Autodesk Inventor part; units mm, degrees
ref_plane "YZ Plane" through (0, 0, 0) normal (1, 0, 0) x (0, 1, 0)
ref_plane "XZ Plane" through (0, 0, 0) normal (0, 1, 0) x (-1, 0, 0)
ref_plane "XY Plane" through (0, 0, 0) normal (0, 0, 1) x (1, 0, 0)
sketch "Sketch2" plane through (0, 0, 0) normal (1, 0, 0) x (0, 1, 0)
  line L0 (0, 0) -> (17, 0)
  line L1 (17, 0) -> (17, -15)
  line L2 (17, -15) -> (0, -15)
  line L3 (0, -15) -> (0, 0)
  dimension "d4" = 17
  dimension "d5" = 15
extrude "Extrusion2" add sketch "Sketch2" along normal blind 165
sketch "Sketch3" plane through (165, 0, 0) normal (1, 0, 0) x (0, 0, -1)
  line L0 (0, 17) -> (0, 0)
  line L1 (0, 0) -> (15, 0)
  line L2 (15, 0) -> (15, 17)
  line L3 (2, 2) -> (13, 2)
  line L4 (13, 2) -> (13, 15)
  line L5 (13, 15) -> (2, 15)
  line L6 (2, 15) -> (2, 2)
  line L7 (2, 2) -> (13, 15) construction
  line L8 (13, 2) -> (2, 15) construction
  point P0 (7.5, 8.5)
  dimension "d9" = 11
  dimension "d10" = 13
extrude "Extrusion3" cut sketch "Sketch3" against normal through all
sketch "Sketch5" plane through (0, 0, -15) normal (0, 0, -1) x (-1, 0, 0)
  line L0 (0, 0) -> (-165, 0)
  line L1 (-165, 0) -> (0, 17)
  line L2 (-165, 0) -> (-165, 17)
  line L3 (0, 0) -> (-165, 17)
  circle A0 centre (-82.5, 8.5) radius 4.5
  dimension "d13" = 9
extrude "Extrusion4" cut sketch "Sketch5" against normal through all contours A0 L1 L3 | L3 L1 A0 | A0 L3 L1 | L3 A0 L1
fillet "Fillet1" radius 1 4 edges at (82.5, 2, -13) (82.5, 2, -2) (82.5, 15, -2) (82.5, 15, -13)
properties part number "caja perfil"
Geometry: final body of the model. Coordinates: model frame, mm. A direction names the side the tool comes from. Give positions to 0.01 mm unless a question says otherwise; leave off trailing zeros. Write each loop counter-clockwise with the first axis right and the second up, starting at its lowest first coordinate (ties: lowest second). Pieces come first, ordered by that corner, then holes. Notation, with made-up numbers: (-20.75, 22.25) -> (-12.75, 22.25) arc R9 cw to (-12.75, 34.25) -> close; hole circle Ø3 at (79, 6.5). An arc over 180 degrees is marked (long way). Answer in a Markdown table with one row per item.
(1) Pin query (flat end, axial travel): pin 1 (8 mm diameter, centred on y = 14.5, z = -10.5, fed in from +X). Return the tip coordinate at first contact, or that it passes through.
Answers below:
| item | result |
|---|---|
| pin 1 | x = 165 |
(2) Draft query along Y for faces 1 (the flat face through (81, 17, -7)), 2 (the flat face through (81, 14, -15)), 3 (the flat face through (84, 4, -2)). Return one class per face: +Y half, -Y half, draft (parallel to the pull), parting line (faces both ways), or undercut.
Answers below:
| item | result |
|---|---|
| face 1 | +Y half |
| face 2 | draft |
| face 3 | undercut |
(3) Section query D-D on x = 28.5. Return loops of the section in (y, z).
Answers below:
| item | result |
|---|---|
| outline | (0, -15) -> (17, -15) -> (17, 0) -> (0, 0) -> close; hole (2, -12) arc R1 ccw to (3, -13) -> (14, -13) arc R1 ccw to (15, -12) -> (15, -3) arc R1 ccw to (14, -2) -> (3, -2) arc R1 ccw to (2, -3) -> close |
(4) Set-up query: faces 4 (the flat face through (0, 8, -1)), 5 (the flat face through (84, 15, -8)). Return all of +Z, -Z, +X, -X, +Y, -Y with unobstructed straight access to the full face (end or side cutting, diameter ignored); none if empty.
Answers below:
| item | result |
|---|---|
| face 4 | +Z, -Z, -X, +Y, -Y |
| face 5 | +X, -X |
(5) Section query B-B on z = -9.75. Return loops of the section in (x, y).
Answers below:
| item | result |
|---|---|
| outline | (0, 0) -> (165, 0) -> (165, 2) -> (0, 2) -> close; (0, 15) -> (165, 15) -> (165, 17) -> (0, 17) -> close |
(6) Ray query, line 1 along Z through (x, y) = (18.5, 4.25); line 2 along Y through (x, z) = (82.5, -0.7); line 3 along X through (y, z) = (8.5, -13.45). Return the intervals inside material, ascending. Write a range as [from, to].
Answers below:
| item | result |
|---|---|
| line 1 | [-15, -13], [-2, 0] |
| line 2 | [0, 4], [13, 17] |
| line 3 | [0, 78], [87, 165] |
(7) Section query A-A on y = 8.5. Return loops of the section in (x, z).
Answers below:
| item | result |
|---|---|
| outline | (0, -15) -> (78, -15) -> (78, -13) -> (0, -13) -> close; (0, -2) -> (78, -2) -> (78, 0) -> (0, 0) -> close; (87, -15) -> (165, -15) -> (165, -13) -> (87, -13) -> close; (87, -2) -> (165, -2) -> (165, 0) -> (87, 0) -> close |
(8) Section query C-C on x = 82.5. Return loops of the section in (y, z), then the cut area to 3 significant figures.
Answers below:
| item | result |
|---|---|
| outline | (0, -15) -> (4, -15) -> (4, -13) -> (3, -13) arc R1 cw to (2, -12) -> (2, -3) arc R1 cw to (3, -2) -> (4, -2) -> (4, 0) -> (0, 0) -> close; (13, -15) -> (17, -15) -> (17, 0) -> (13, 0) -> (13, -2) -> (14, -2) arc R1 cw to (15, -3) -> (15, -12) arc R1 cw to (14, -13) -> (13, -13) -> close |
| area | 76.9 mm^2 |
